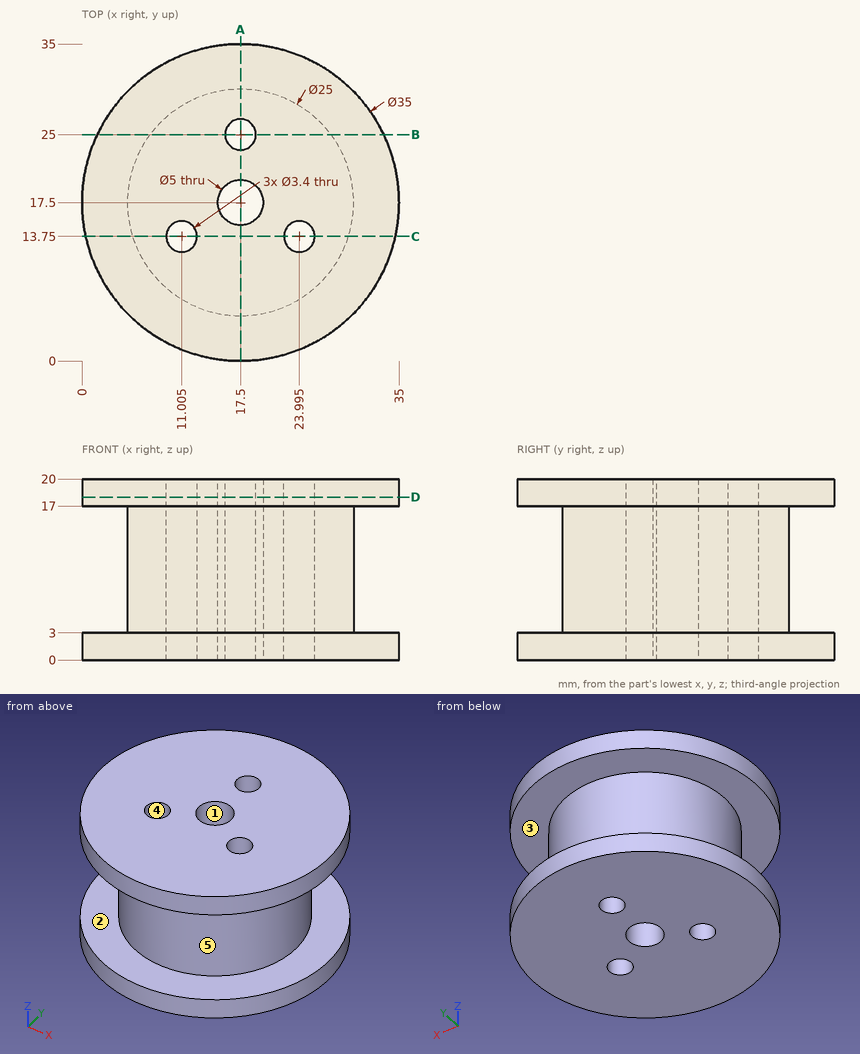
Input: dimensioned drawing with shaded views. Units: mm. Origin: part minimum x, y, z. A direction names the side the tool comes from. Give positions to 0.01 mm unless a question says otherwise; leave off trailing zeros. Write each loop counter-clockwise with the first axis right and the second up, starting at its lowest first coordinate (ties: lowest second). Pieces come first, ordered by that corner, then holes. Notation, with made-up numbers: (-20.5, 32.25) - (-11.5, 32.25) arc R23 cw to (-11.5, 62.25) - close; hole circle Ø9 at (54, -4). An arc over 180 degrees is marked (long way). Write item = value, one per line. Start each with the question number.
1) Pin query (flat end, axial travel): pin 1 (1 mm diameter, centred on y = 18.5, z = 8, fed in from +X); pin 2 (12 mm diameter, centred on y = 20, z = 11.5, fed in from +X); pin 3 (1.5 mm diameter, centred on x = 29.5, z = 12.5, fed in from -Y). Return the tip coordinate at first contact, or that it passes through.
2) Cut plane A-A (x = 17.5). Return loops of the section in (y, z).
3) Reachability of the marked faces 1 and 2 from +Z, -Z, +X, -X, +Y, -Y: full face, straight path, thin tool, end or side. Return the list, or none.
4) Cut plane D-D (z = 18). Give the number of separate pieces and of enclosed holes in the cut face, and give its area (3 significant figures).
5) Draft query along X for the marked faces 3, 4 and 5. Return one class per face: pulls with the +X half, pulls with the -X half, needs draft (parallel to the pull), parting line crosses it, or undercut.
6) Cut plane C-C (y = 13.75). Return loops of the section in (x, z) (1 decimal).
7) Material intervals for L1, parallel to Y at x = 17.5, z = 6.5; L2, parallel to Z at x = 31, y = 19; L3, parallel to X at y = 26, z = 2 (1 decimal), sorted ascending. Write a range as [from, to].
8) Cut plane B-B (y = 25). Return loops of the section in (x, z).
Answers follow:
q1.pin_1 = 29.99
q1.pin_2 = 35
q1.pin_3 = 12.05
q2.outline = (0, 0) - (15, 0) - (15, 20) - (0, 20) - (0, 17) - (5, 17) - (5, 3) - (0, 3) - close; (20, 0) - (23.3, 0) - (23.3, 20) - (20, 20) - close; (26.7, 0) - (35, 0) - (35, 3) - (30, 3) - (30, 17) - (35, 17) - (35, 20) - (26.7, 20) - close
q3.face_1 = +Z, -Z
q3.face_2 = none
q4.separate_pieces = 1
q4.enclosed_holes = 4
q4.area = 915 mm^2
q5.face_3 = needs draft
q5.face_4 = undercut
q5.face_5 = parting line crosses it
q6.outline = (0.4, 0) - (9.3, 0) - (9.3, 20) - (0.4, 20) - (0.4, 17) - (5.6, 17) - (5.6, 3) - (0.4, 3) - close; (12.7, 0) - (22.3, 0) - (22.3, 20) - (12.7, 20) - close; (25.7, 0) - (34.6, 0) - (34.6, 3) - (29.4, 3) - (29.4, 17) - (34.6, 17) - (34.6, 20) - (25.7, 20) - close
q7.L1 = [5, 15], [20, 23.3], [26.7, 30]
q7.L2 = [0, 3], [17, 20]
q7.L3 = [2.2, 16.1], [18.9, 32.8]
q8.outline = (1.69, 0) - (15.8, 0) - (15.8, 20) - (1.69, 20) - (1.69, 17) - (7.5, 17) - (7.5, 3) - (1.69, 3) - close; (19.2, 0) - (33.31, 0) - (33.31, 3) - (27.5, 3) - (27.5, 17) - (33.31, 17) - (33.31, 20) - (19.2, 20) - close
